from build123d import *

# Parameters (mm, degrees)
SKETCH1_R           = 2.1
BOSS_EXTRUDE1_DEPTH = 65
BOSS_EXTRUDE6_DEPTH = 200
SKETCH85_W          = 34.906324044
SKETCH85_H          = 40.252337635
CUT_EXTRUDE59_DEPTH = 65
SKETCH87_W          = 20
SKETCH87_H          = 15
BOSS_EXTRUDE7_DEPTH = 11
SKETCH88_W          = 1.985779144
SKETCH88_H          = 1.348664344
SKETCH88_W_2        = 1.884447459
SKETCH88_H_2        = 1.174834559
CUT_EXTRUDE60_DEPTH = 11
CUT_EXTRUDE61_DEPTH = 189


with BuildPart() as part:
    # Sketch1 → Boss-Extrude1 (new body)
    with BuildSketch(Plane(origin=(0, 0, 0), x_dir=(0, 0, -1), z_dir=(1, 0, 0))):
        with BuildLine():
            Line((-10, 9), (-10, 3))
            Line((-10, 3), (-8, 3))
            Line((-8, 3), (-8, 6))
            Line((-8, 6), (-7.060660172, 6))
            Line((-7.060660172, 6), (-4, 2.939339828))
            Line((-4, 2.939339828), (-4, -2.939339828))
            Line((-4, -2.939339828), (-7.060660172, -6))
            Line((-7.060660172, -6), (-8, -6))
            Line((-8, -6), (-8, -3))
            Line((-8, -3), (-10, -3))
            Line((-10, -3), (-10, -9))
            ThreePointArc((-10, -9), (-9.707106781, -9.707106781), (-9, -10))
            Line((-9, -10), (-3, -10))
            Line((-3, -10), (-3, -8))
            Line((-3, -8), (-6, -8))
            Line((-6, -8), (-6, -7.060660172))
            Line((-6, -7.060660172), (-2.939339828, -4))
            Line((-2.939339828, -4), (2.939339828, -4))
            Line((2.939339828, -4), (6, -7.060660172))
            Line((6, -7.060660172), (6, -8))
            Line((6, -8), (3, -8))
            Line((3, -8), (3, -10))
            Line((3, -10), (9, -10))
            ThreePointArc((9, -10), (9.707106781, -9.707106781), (10, -9))
            Line((10, -9), (10, -3))
            Line((10, -3), (8, -3))
            Line((8, -3), (8, -6))
            Line((8, -6), (7.060660172, -6))
            Line((7.060660172, -6), (4, -2.939339828))
            Line((4, -2.939339828), (4, 2.939339828))
            Line((4, 2.939339828), (7.060660172, 6))
            Line((7.060660172, 6), (8, 6))
            Line((8, 6), (8, 3))
            Line((8, 3), (10, 3))
            Line((10, 3), (10, 9))
            ThreePointArc((10, 9), (9.707106781, 9.707106781), (9, 10))
            Line((9, 10), (3, 10))
            Line((3, 10), (3, 8))
            Line((3, 8), (6, 8))
            Line((6, 8), (6, 7.060660172))
            Line((6, 7.060660172), (2.939339828, 4))
            Line((2.939339828, 4), (-2.939339828, 4))
            Line((-2.939339828, 4), (-6, 7.060660172))
            Line((-6, 7.060660172), (-6, 8))
            Line((-6, 8), (-3, 8))
            Line((-3, 8), (-3, 10))
            Line((-3, 10), (-9, 10))
            ThreePointArc((-9, 10), (-9.707106781, 9.707106781), (-10, 9))
        make_face()
        Circle(SKETCH1_R, mode=Mode.SUBTRACT)
    extrude(amount=BOSS_EXTRUDE1_DEPTH)

    # Sketch85 → Cut-Extrude59 (cut)
    with BuildSketch(Plane.ZY):
        with Locations((-1.630437185, 0.066948306)):
            Rectangle(SKETCH85_W, SKETCH85_H)
    extrude(amount=-CUT_EXTRUDE59_DEPTH, mode=Mode.SUBTRACT)


with BuildPart() as body_2:
    # Sketch84 → Boss-Extrude6 (new body)
    with BuildSketch(Plane(origin=(65, 0, 0), x_dir=(0, 0, -1), z_dir=(1, 0, 0))):
        Polygon((-150, -2.9), (-150, 2.9), (-152.1, 2.9), (-152.1, 5.9), (-152.897918472, 5.9), (-155.9, 2.897918472), (-155.9, -2.897918472), (-152.897918472, -5.9), (-152.1, -5.9), (-152.1, -2.9), align=None)
        Polygon((-80, -10), (-80, 5), (-150, 5), (-150, 3), (-150, 2.9), (-150, -2.9), (-150, -3), (-150, -10), align=None)
        Polygon((-10, 2.9), (-10, 3), (-10, 5), (-80, 5), (-80, -10), (-10, -10), (-10, -9), (-10, -3), (-10, -2.9), (-7.9, -2.9), (-7.9, -5.9), (-7.102081528, -5.9), (-4.1, -2.897918472), (-4.1, 2.897918472), (-7.102081528, 5.9), (-7.9, 5.9), (-7.9, 2.9), align=None)
    extrude(amount=BOSS_EXTRUDE6_DEPTH)

    # Sketch87 → Boss-Extrude7 (add)
    with BuildSketch(Plane.ZY.offset(-65)):
        with Locations((160, -2.5)):
            Rectangle(SKETCH87_W, SKETCH87_H)
        with Locations((0, -2.5)):
            Rectangle(SKETCH87_W, SKETCH87_H)
    extrude(amount=-BOSS_EXTRUDE7_DEPTH)

    # Sketch88 → Cut-Extrude60 (cut)
    with BuildSketch(Plane.ZY.offset(-65)):
        with Locations((153.092889572, 5.674332172)):
            Rectangle(SKETCH88_W, SKETCH88_H)
        with Locations((6.957776271, 5.58741728)):
            Rectangle(SKETCH88_W_2, SKETCH88_H_2)
    extrude(amount=-CUT_EXTRUDE60_DEPTH, mode=Mode.SUBTRACT)

    # Sketch89 → Cut-Extrude61 (cut)
    with BuildSketch(Plane(origin=(265, 0, 0), x_dir=(0, 0, -1), z_dir=(1, 0, 0))):
        Polygon((-7.9, 2.9), (-10, 2.9), (-10, 2.5), (-9.6, 2.5), (-7.5, 2.5), (-7.5, 5.5), (-7.267766953, 5.5), (-4.5, 2.732233047), (-4.5, -2.732233047), (-7.267766953, -5.5), (-7.5, -5.5), (-7.5, -2.5), (-9.6, -2.5), (-10, -2.5), (-10, -2.9), (-7.9, -2.9), (-7.9, -5.9), (-7.102081528, -5.9), (-4.1, -2.897918472), (-4.1, 2.897918472), (-7.102081528, 5.9), (-7.9, 5.9), align=None)
        Polygon((-150, 2.5), (-150, 2.9), (-152.1, 2.9), (-152.1, 5.9), (-152.897918472, 5.9), (-155.9, 2.897918472), (-155.9, -2.897918472), (-152.897918472, -5.9), (-152.1, -5.9), (-152.1, -2.9), (-150, -2.9), (-150, -2.5), (-150.4, -2.5), (-152.5, -2.5), (-152.5, -5.5), (-152.732233047, -5.5), (-155.5, -2.732233047), (-155.5, 2.732233047), (-152.732233047, 5.5), (-152.5, 5.5), (-152.5, 2.5), (-150.4, 2.5), align=None)
    extrude(amount=-CUT_EXTRUDE61_DEPTH, mode=Mode.SUBTRACT)


solid = body_2.part
Work out the finished part from the listing and answer in its coordinate system (mm). A direction names the side the tool comes from. Round coordinates to 2 decimals unless told otherwise and drop trailing zeros. Loops run counter-clockwise (first coordinate to the right, second up) from the corner with the lowest first, then second, coordinate; pieces in that order, holes last. Notation, with made-up numbers: M 46,-24.5 L 51,-24.5 A20 ccw 51,13.5 Z; hole C -37.75,10.25 d8. An arc over 180 degrees is marked long. One line per question, with ' | ' between items. Start each with the question number.
(1) A cutting plane is placed at B-B on x = 84.5. Write down the section's boundary in (y, z), plus the area to 3 significant figures.
(2) A tool of negligible diameter and unlimited length cuts with its end or side. For faces 5 (the face through (164, -10, 79)), 6 (the face through (164, 5, 79)), 7 (the face through (169, -6, 10)), from which of +Z, -Z, +X, -X, +Y, -Y can it reach the whole face along a straight path? Write none if from no direction.
(3) A cutting plane is placed at A-A on y = 0. Write down the section's boundary in (x, z), plus the area to 3 significant figures.
(4) Find the intervals of material crossed by line 1 (Z direction, x = 184.5, y = -5); line 2 (Z direction, x = 81.5, y = 3); line 3 (Z direction, x = 116, y = -9), in increasing order.
(5) For a pull along Z with two mould halves and no side action, classify faces 1 (the face through (65, -2, 79)), 2 (the face through (169, -6, 150)), 3 (the face through (172, 0, 155.5)), 4 (the face through (172, 0, 4.5)) as released by +Z, released by -Z, zero draft, split by the parting line, or undercut.
(6) A cutting plane is placed at C-C on z = 38. Write down the section's boundary in (x, y), plus the area to 3 significant figures.
(7) Flat-ended cylindrical pins translate along their axes: pin 1 Ø12 at (x, z) = (184.5, 43) entering from +Y; pin 2 Ø5 at (x, y) = (200.5, -5) entering from +Z; pin 3 Ø8 at (x, y) = (170, -6) entering from -Z. Find the tip coordinate at first contact, or state that the pin passes through.
Geometry check:
1) outline: M -10,10 L -2.5,10 L -2.5,7.5 L -5.5,7.5 L -5.5,7.27 L -2.73,4.5 L 2.73,4.5 L 5.5,7.27 L 5.5,7.5 L 2.5,7.5 L 2.5,10 L 5,10 L 5,150 L 2.5,150 L 2.5,152.5 L 5.5,152.5 L 5.5,152.73 L 2.73,155.5 L -2.73,155.5 L -5.5,152.73 L -5.5,152.5 L -2.5,152.5 L -2.5,150 L -10,150 Z | area: 2,180 mm²
2) face 5: +Z, -Z, +X, -X, -Y | face 6: +X, -X, +Y | face 7: +X, -Y
3) outline: M 65,-10 L 76,-10 L 76,4.5 L 265,4.5 L 265,155.5 L 76,155.5 L 76,170 L 65,170 Z | area: 30,500 mm²
4) line 1: z = 6.77 to 7.5, 10 to 150, 152.5 to 153.23 | line 2: z = 4.77 to 7.5, 10 to 150, 152.5 to 155.23 | line 3: z = 10 to 150
5) face 1: zero draft | face 2: undercut | face 3: released by +Z | face 4: released by -Z
6) outline: M 65,-10 L 265,-10 L 265,5 L 65,5 Z | area: 3,000 mm²
7) pin 1: stops at y = 5 | pin 2: stops at z = 155.5 | pin 3: stops at z = 4.5
